Geometry check sheet. Reference: drawing and pictorial views, mm from the part's lowest x, y, z. A direction names the side the tool comes from. Round coordinates to 2 decimals unless told otherwise and drop trailing zeros. Order: outer loops, then holes, each group sorted by start corner. A loop starts at its lowest first (then second) coordinate and runs counter-clockwise, first axis right, second up.
(1) Sectioned sample at C-C, the plane y = 7. Enter the section's corners in (x, z).
(2) Sectioned sample at A-A, the plane x = 53. Enter the section's corners in (y, z), and give its area (3 significant figures).
(3) Depth check by flat-ended pin: pin 1 (5 mm diameter, centred on x = 22, z = 16, fed in from +Y). Enter the tip coordinate at first touch or a pass-through.
(4) Sectioned sample at B-B, the plane z = 22.5. Enter the section's corners in (x, y), and give its area (3 significant figures).
(5) Thickness scan on probe 1 along Y at (x, z) = (29, 23); probe 2 along Z at (x, y) = (44, 28.5). Record the ranges inside material, lowest first.
(6) Tool access check on the marked faces 1 and 2. Record the directions out of +Z, -Z, +X, -X, +Y, -Y that give a thin tool (end or side, any length) a straight path to the whole face; none if there is none.
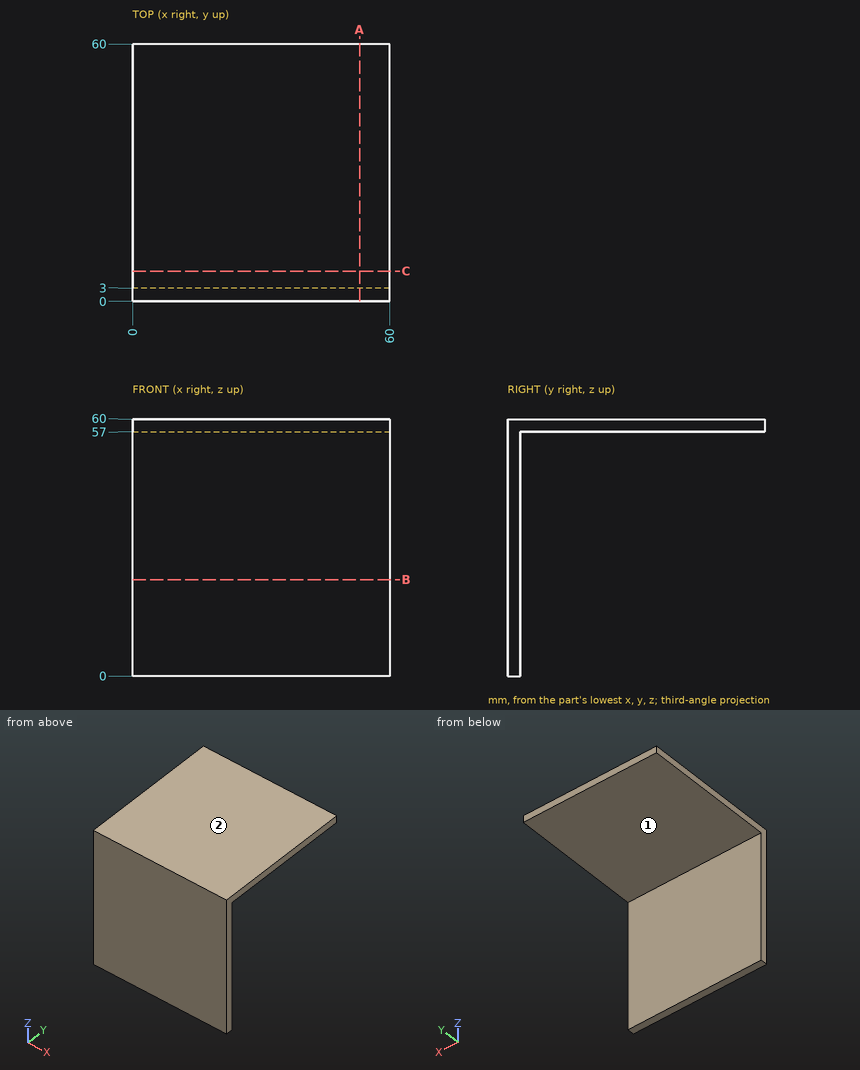
Derived:
1. outline: (0, 57) - (60, 57) - (60, 60) - (0, 60) - close
2. outline: (0, 0) - (3, 0) - (3, 57) - (60, 57) - (60, 60) - (0, 60) - close
2. area: 351 mm2
3. pin 1: stops at y = 3
4. outline: (0, 0) - (60, 0) - (60, 3) - (0, 3) - close
4. area: 180 mm2
5. probe 1: y = 0 to 3
5. probe 2: z = 57 to 60
6. face 1: -Z, +X, -X, +Y
6. face 2: +Z, +X, -X, +Y, -Y
